For this review, take the finished solid that the model builds, in its own axes (mm). Face numbers are marked on the shaded views. Coordinates: 2 decimals unless noted, no trailing zeros. Write each loop counter-clockwise with the first axis right and the second up, starting at its lowest first coordinate (ties: lowest second). Pieces come first, ordered by that corner, then holes.
1) Insertion check: P1, Ø1.5, axis at x = 6.5, y = -8, coming from the -Z side. The pin has a flat end and moves straight along its axis. Give the tip position at first contact, or say it passes through.
2) We need section C-C on y = -10. Write out the cut boundary in (x, z) (3 decimals), then the cut area to 3 significant figures.
3) We need section B-B on x = 30. Write out the cut boundary in (y, z), then the cut area to 3 significant figures.
4) Mouldability with a two-part tool opening along Z and no side actions: class the marked faces 1, 2 and 3 as pulls with the +Z half, pulls with the -Z half, needs draft (parallel to the pull), parting line crosses it, or undercut.
5) To check wall thickness, follow line 1 along Y through (x, z) = (30, 6.5); line 2 along Y through (x, z) = (-29, 1.5); line 3 along Z through (x, y) = (-6.5, 9.5). State the ranges of each line that lie inside material, in increasing order.
6) We need section A-A on z = 17. Write out the cut boundary in (x, y), then the cut area to 3 significant figures.
7) We need section D-D on z = 1.5. Write out the cut boundary in (x, y), then the cut area to 3 significant figures.
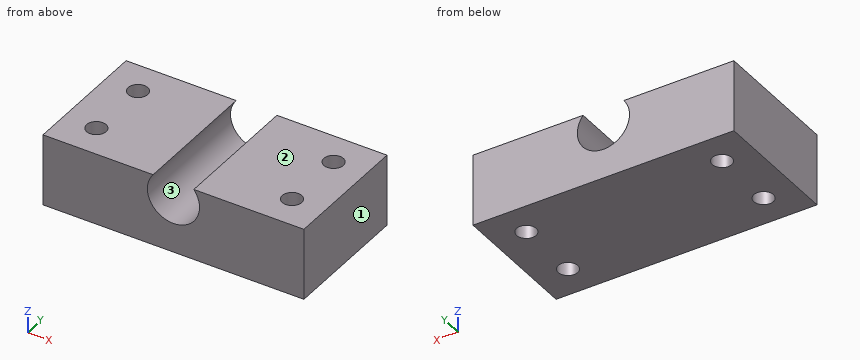
from build123d import *

# Parameters (mm, degrees)
SCHIZZO1_W                   = 80
SCHIZZO1_H                   = 40
ESTRUSIONE_ESTRUSIONE1_DEPTH = 22
SCHIZZO2_R                   = 8
TAGLIO_ESTRUSIONE1_DEPTH     = 61.695963622
SCHIZZO3_R                   = 3
TAGLIO_ESTRUSIONE2_DEPTH     = 50.839743178


with BuildPart() as part:
    # Schizzo1 → Estrusione-Estrusione1 (new body)
    with BuildSketch(Plane.XY):
        Rectangle(SCHIZZO1_W, SCHIZZO1_H)
    extrude(amount=ESTRUSIONE_ESTRUSIONE1_DEPTH)

    # Schizzo2 → Taglio-Estrusione1 (cut, through all)
    with BuildSketch(Plane.XZ.offset(20)):
        with Locations((0, 17)):
            Circle(SCHIZZO2_R)
    extrude(amount=-TAGLIO_ESTRUSIONE1_DEPTH, mode=Mode.SUBTRACT)

    # Schizzo3 → Taglio-Estrusione2 (cut, through all)
    with BuildSketch(Plane.XY.offset(22)):
        with Locations((-30, 10)):
            Circle(SCHIZZO3_R)
        with Locations(Location((-30, -10, 0), (0, 0, 180))):
            Circle(SCHIZZO3_R)
        with Locations((30, -10)):
            Circle(SCHIZZO3_R)
        with Locations(Location((30, 10, 0), (0, 0, 180))):
            Circle(SCHIZZO3_R)
    extrude(amount=-TAGLIO_ESTRUSIONE2_DEPTH, mode=Mode.SUBTRACT)


solid = part.part
Result:
1. P1: stops at z = 0
2. outline: (-40, 0) - (-33, 0) - (-33, 22) - (-40, 22) - close; (-27, 0) - (27, 0) - (27, 22) - (6.245, 22) arc R8 cw (long way) to (-6.245, 22) - (-27, 22) - close; (33, 0) - (40, 0) - (40, 22) - (33, 22) - close
2. area: 1,320 mm2
3. outline: (-20, 0) - (-13, 0) - (-13, 22) - (-20, 22) - close; (-7, 0) - (7, 0) - (7, 22) - (-7, 22) - close; (13, 0) - (20, 0) - (20, 22) - (13, 22) - close
3. area: 616 mm2
4. face 1: needs draft
4. face 2: pulls with the +Z half
4. face 3: undercut
5. line 1: y = -20 to -13, -7 to 7, 13 to 20
5. line 2: y = -20 to -12.83, -7.17 to 7.17, 12.83 to 20
5. line 3: z = 0 to 12.34, 21.66 to 22
6. outline: (-40, -20) - (-8, -20) - (-8, 20) - (-40, 20) - close; (8, -20) - (40, -20) - (40, 20) - (8, 20) - close; hole circle Ø6 at (-30, -10); hole circle Ø6 at (-30, 10); hole circle Ø6 at (30, -10); hole circle Ø6 at (30, 10)
6. area: 2,450 mm2
7. outline: (-40, -20) - (40, -20) - (40, 20) - (-40, 20) - close; hole circle Ø6 at (-30, -10); hole circle Ø6 at (-30, 10); hole circle Ø6 at (30, -10); hole circle Ø6 at (30, 10)
7. area: 3,090 mm2
